Job drawing, mm, ordinate dimensions from the low corner. One solid piece. A direction names the side the tool comes from. Coordinates: 2 decimals unless noted, no trailing zeros. Loops run counter-clockwise (first coordinate to the right, second up) from the corner with the lowest first, then second, coordinate; pieces in that order, holes last. Notation, with made-up numbers: (21, -20.75) -> (39, -20.75) arc R12 ccw to (39, -10.75) -> close; hole circle Ø11 at (22.25, 63). An arc over 180 degrees is marked (long way). Use one line per item in the form item = value. Start each with the question number.
(1) Band-saw the part on B-B on z = 107. Give the cut face in (x, y), then the cut area to 3 significant figures.
(2) Band-saw the part on A-A on y = 7. Give the cut face in (x, z), then the cut area to 3 significant figures.
(3) Mould opens along Z. For the marked faces 4, 5 and 6 say: +Z half, -Z half, draft (parallel to the pull), parting line (faces both ways), or undercut.
(4) Band-saw the part on D-D on z = 38.5. Give the cut face in (x, y).
(5) Band-saw the part on C-C on y = 23.5. Give the cut face in (x, z), then the cut area to 3 significant figures.
(6) Pin check, flat tips, straight feed: P1, Ø4, axis at y = 22, z = 92, coming from the +X side (1 decimal); P2, Ø5, axis at x = 51.5, z = 47, coming from the +Y side; P3, Ø1, axis at x = 21, z = 65, coming from the -Y side (1 decimal). Stop position of each tip, or through.
(7) Drill centre lines: L1, parallel to Z at x = 38, y = 7; L2, parallel to Z at x = 40, y = 17; L3, parallel to Y at x = 50, z = 61.5. Where is each one in solid material? Low to high. Write a range as [from, to].
(8) 3-axis set-ups, long thin cutter, end or side, ignore diameter. For the marked faces 1, 2 and 3: which of +Z, -Z, +X, -X, +Y, -Y reach the whole face in a straight line?
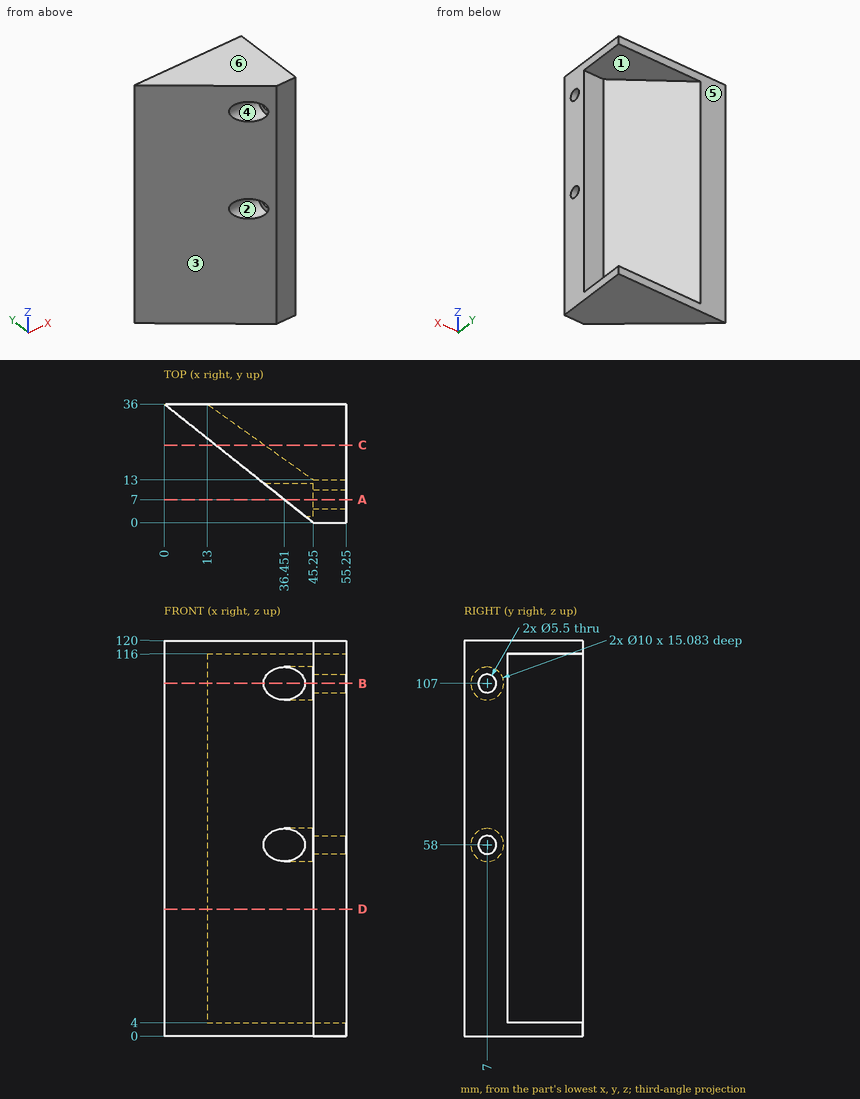
A:
q1.outline = (0, 36) -> (30.17, 12) -> (45.25, 12) -> (45.25, 9.75) -> (55.25, 9.75) -> (55.25, 13) -> (45.25, 13) -> (13, 36) -> close; (42.74, 2) -> (45.25, 0) -> (55.25, 0) -> (55.25, 4.25) -> (45.25, 4.25) -> (45.25, 2) -> close
q1.area = 431 mm²
q2.outline = (36.45, 0) -> (55.25, 0) -> (55.25, 55.25) -> (45.25, 55.25) -> (45.25, 53) -> (36.45, 53) -> close; (36.45, 63) -> (45.25, 63) -> (45.25, 60.75) -> (55.25, 60.75) -> (55.25, 104.25) -> (45.25, 104.25) -> (45.25, 102) -> (36.45, 102) -> close; (36.45, 112) -> (45.25, 112) -> (45.25, 109.75) -> (55.25, 109.75) -> (55.25, 120) -> (36.45, 120) -> close
q2.area = 1,970 mm²
q3.face_4 = undercut
q3.face_5 = draft
q3.face_6 = +Z half
q4.outline = (0, 36) -> (45.25, 0) -> (55.25, 0) -> (55.25, 13) -> (45.25, 13) -> (13, 36) -> close
q5.outline = (15.71, 0) -> (55.25, 0) -> (55.25, 4) -> (30.53, 4) -> (30.53, 116) -> (55.25, 116) -> (55.25, 120) -> (15.71, 120) -> close
q5.area = 1,980 mm²
q6.P1 = 35.4
q6.P2 = 13
q6.P3 = 18.9
q7.L1 = [0, 53], [63, 102], [112, 120]
q7.L2 = [0, 4], [116, 120]
q7.L3 = [0, 13]
q8.face_1 = +X, +Y
q8.face_2 = -X
q8.face_3 = +Z, -Z, -X, -Y
